```python
from build123d import *

# Parameters (mm, degrees)
SKETCH_1_W          = 1915
SKETCH_1_H          = 80
EXTRUDE_1_DEPTH     = 80
SKETCH_3_W          = 68
SKETCH_3_H          = 68
CUT_EXTRUDE_2_DEPTH = 1919.339125389


with BuildPart() as part:
    # 草图1 → 拉伸1 (new body)
    with BuildSketch(Plane.XY):
        with Locations((957.5, 40)):
            Rectangle(SKETCH_1_W, SKETCH_1_H)
    extrude(amount=EXTRUDE_1_DEPTH)

    # 草图3 → 拉伸2 (cut, through all)
    with BuildSketch(Plane.ZY):
        with Locations((46, 46)):
            Rectangle(SKETCH_3_W, SKETCH_3_H)
    extrude(amount=-CUT_EXTRUDE_2_DEPTH, mode=Mode.SUBTRACT)


solid = part.part
```
Here's how the part is built. I have some questions about the finished solid (model axes, mm). A direction names the side the tool comes from. Coordinates: 2 decimals unless noted, no trailing zeros. Order: outer loops, then holes, each group sorted by start corner. A loop starts at its lowest first (then second) coordinate and runs counter-clockwise, first axis right, second up. Notation, with made-up numbers: M 88.25,-29 L 121.25,-29 A26 cw 121.25,4 Z; hole C 50,41.25 d6. An arc over 180 degrees is marked long. Answer as a JSON object with one key per item and string values. Group by question number.
(1) Suppose I cut it at B-B, the plane y = 68. Please give me the cut outline in (x, z), then the cut area to 3 significant figures.
(2) For pin 1 (1.5 mm diameter, centred on x = 260.5, y = 66, fed in from +Z), with a flat end and sliding along its axis, tell me the tip position at first contact or that it passes through.
(3) Suppose I cut it at A-A, the plane x = 724.5. Please give me the cut outline in (y, z).
(4) Which directions (+Z, -Z, +X, -X, +Y, -Y) give clear straight access to the entire face, cutting with the end or side of a thin tool? Please do faces 1 (the face through (944, 46, 12)), 2 (the face through (944, 41, 0)).
(5) I need wall thicknesses on probe 1 along Y at (x, z) = (1498, 32). Which ranges of the line are inside material? Lowest first, please.
Values found:
{
 "1": {"outline": "M 0,0 L 1915,0 L 1915,12 L 0,12 Z", "area": "23,000 mm^2"},
 "2": {"pin 1": "stops at z = 12"},
 "3": {"outline": "M 0,0 L 80,0 L 80,12 L 12,12 L 12,80 L 0,80 Z"},
 "4": {"face 1": "+Z, +X, -X, +Y", "face 2": "-Z, +X, -X, +Y, -Y"},
 "5": {"probe 1": "y = 0 to 12"}
}
